Autodesk Inventor part; units mm, degrees
ref_plane "YZ Plane" through (0, 0, 0) normal (1, 0, 0) x (0, 1, 0)
ref_plane "XZ Plane" through (0, 0, 0) normal (0, 1, 0) x (-1, 0, 0)
ref_plane "XY Plane" through (0, 0, 0) normal (0, 0, 1) x (1, 0, 0)
sketch "Sketch1" plane through (0, 0, 0) normal (0, 1, 0) x (-1, 0, 0)
  circle A0 centre (0, 0) radius 3
  dimension "d0" = 6
extrude "Extrusion1" add sketch "Sketch1" along normal blind 70
sketch "Sketch2" plane through (0, 70, 0) normal (0, 1, 0) x (1, 0, 0)
  point P0 (0, 0)
sketch "Sketch3" plane through (0, 0, 0) normal (1, 0, 0) x (0, 1, 0)
  line L0 (0, 0) -> (0, -9)
  line L1 (0, -3) -> (0, 3)
  line L2 (0, 0) -> (-9, 0)
  arc A0 (-9, 0) -> (0, -9) centre (0, 0) ccw
  line L3 (70, -3) -> (70, 3)
  arc A1 (70, -9) -> (79, 0) centre (70, 0) ccw
  line L4 (79, 0) -> (70, 0)
  line L5 (70, -9) -> (70, 0)
  dimension "d3" = 9
  dimension "d4" = 9
  dimension "d5" = 9
revolve "Revolution1" add sketch "Sketch3" angle 360 about axis through (0, 79, 0) along (0, -1, 0)
sketch "Sketch4" plane through (0, 0, 0) normal (1, 0, 0) x (0, 1, 0)
  line L0 (0, -10.1336) -> (-13.8396, -10.1336)
  line L1 (-13.8396, -10.1336) -> (-13.8396, 13.3764)
  line L2 (-13.8396, 13.3764) -> (0, 13.3764)
  line L3 (0, 13.3764) -> (0, -10.1336)
  line L4 (70, 9) -> (70, -9)
  line L5 (70, -9) -> (70, 12.4499)
  line L6 (70, 12.4499) -> (83.9063, 12.4499)
  line L7 (83.9063, 12.4499) -> (83.9063, -12.3341)
  line L8 (83.9063, -12.3341) -> (70, -9)
  point P0 (0, 0)
extrude "Extrusion2" cut sketch "Sketch4" along normal mid plane 20
sketch "Sketch5" plane through (0, 0, 0) normal (1, 0, 0) x (0, 1, 0)
  line L0 (0, 0) -> (0, -6)
  line L1 (0, -3) -> (0, 3)
  line L2 (0, 0) -> (-6, 0)
  arc A0 (-6, 0) -> (0, -6) centre (0, 0) ccw
  line L3 (70, -3) -> (70, 3)
  line L4 (70, 0) -> (76, 0)
  line L5 (70, 0) -> (70, -6)
  arc A1 (70, -6) -> (76, 0) centre (70, 0) ccw
  dimension "d9" = 6
  dimension "d10" = 6
  dimension "d11" = 6
  dimension "d12" = 6
revolve "Revolution2" add sketch "Sketch5" angle 360 about axis through (0, 70, 0) along (0, 1, 0)
properties part number "Pino da dobradiça"
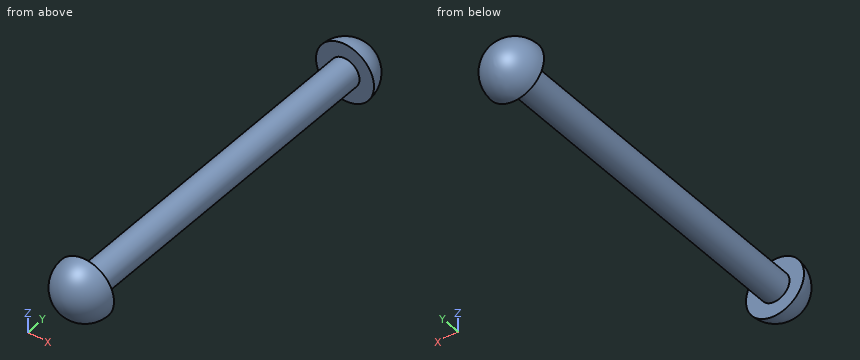
Design review of the part built by this model. Coordinates are the model's own, in mm. Give positions to 0.01 mm unless a question says otherwise; leave off trailing zeros. Order: outer loops, then holes, each group sorted by start corner. A loop starts at its lowest first (then second) coordinate and runs counter-clockwise, first axis right, second up. Notation, with made-up numbers: (32.5, 70) - (89.5, 70) arc R32 ccw to (89.5, 100) - close; hole circle Ø11 at (72.5, -21). An arc over 180 degrees is marked (long way). Use a Markdown table: item, result. Add a question column.
(1) Add section D-D on y = 12. Give the boundary of the cut face in (x, z).
(2) Add section C-C on x = -4. Give the boundary of the cut face in (y, z), then the cut area to 3 significant figures.
(3) Clearance check with flat-ended pins moving along their axes: P1, Ø2, axis at x = -1.5, y = 56.5, coming from the +Z side; P2, Ø2, axis at y = 46.5, z = -2, coming from the -X side; P3, Ø3.5, axis at x = -0.5, z = 2.5, coming from the +Y side. State where each tip first meets the part, or that it passes through.
(4) Add section B-B on z = 0. Give the boundary of the cut face in (x, y).
(5) Add section A-A on x = 0. Give the boundary of the cut face in (y, z).
(6) Wall thickness on probe 1 along Z at (x, y) = (-0.25, 9); probe 2 along Y at (x, z) = (-1.25, 4): over which ranges is each line inside the solid? List them lowest first. Write a range as [from, to].
Report:
| question | item | result |
|---|---|---|
| 1 | outline | circle Ø6 at (0, 0) |
| 2 | outline | (0, -4.47) - (0, 4.47) arc R4.47 ccw to start; (70, -4.47) arc R4.47 ccw to (70, 4.47) - close |
| 2 | area | 62.8 mm² |
| 3 | P1 | stops at z = 2.96 |
| 3 | P2 | stops at x = -2.83 |
| 3 | P3 | stops at y = 75.95 |
| 4 | outline | (-6, 0) arc R6 ccw to (6, 0) - (3, 0) - (3, 70) - (6, 70) arc R6 ccw to (-6, 70) - (-3, 70) - (-3, 0) - close |
| 5 | outline | (0, -6) - (0, -3) - (70, -3) - (70, -6) arc R6 ccw to (70, 6) - (70, 3) - (0, 3) - (0, 6) arc R6 ccw to start |
| 6 | probe 1 | z = [-2.99, 2.99] |
| 6 | probe 2 | y = [-4.29, 0], [70, 74.29] |
